The figure shows three views and two pictorial views of one solid part (mm, origin at its lowest corner). Answer the questions. Coordinates: 2 decimals unless noted, no trailing zeros. Write each loop counter-clockwise with the first axis right and the second up, starting at its lowest first coordinate (ties: lowest second). Pieces come first, ordered by that corner, then holes. Notation, with made-up numbers: M 70.5,85.5 L 99.5,85.5 A14 ccw 99.5,108.5 Z; hole C 81.5,-36 d10. An arc over 180 degrees is marked long. Write item = value, one per line.
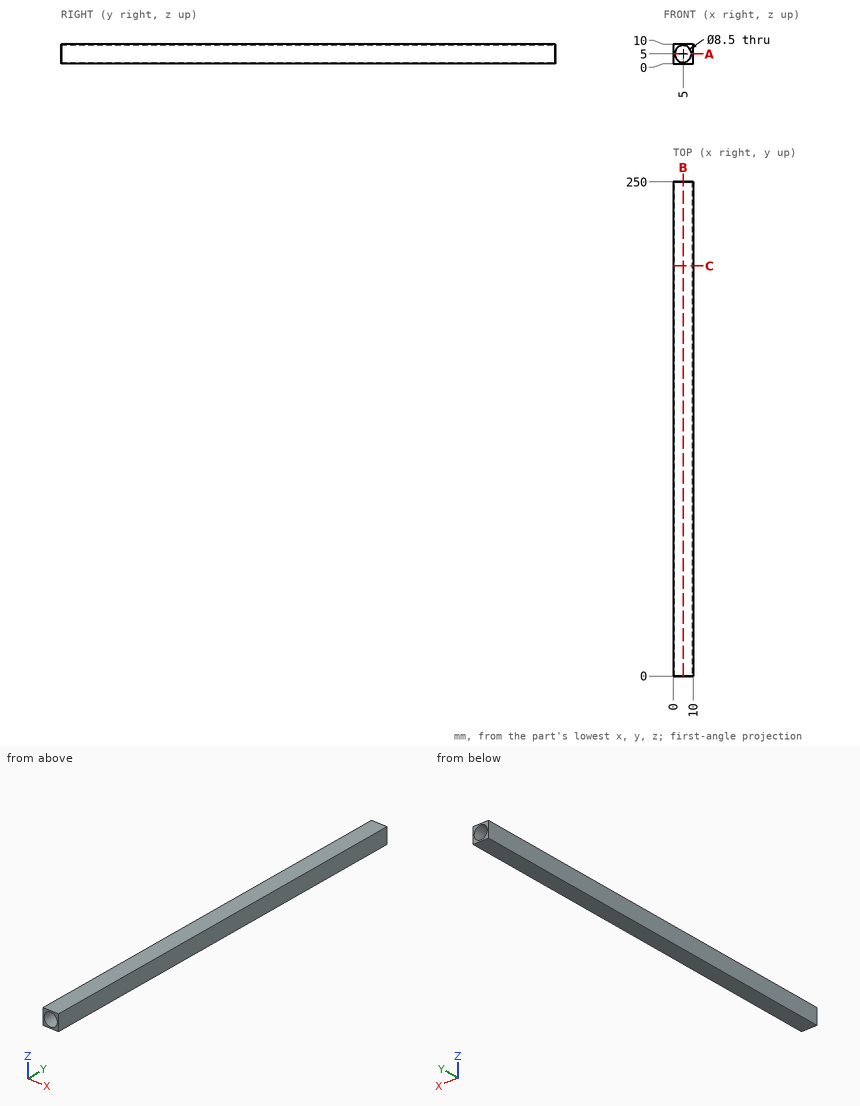
Item 1: Consider line 1 along Z through (x, y) = (5.5, 35); line 2 along X through (y, z) = (232, 8.5); line 3 along Z through (x, y) = (3.75, 213). Determine where each line is inside the solid, lowest interval first. Write a range as from..to.
Worked answers:
line_1 = 0..0.78, 9.22..10
line_2 = 0..2.59, 7.41..10
line_3 = 0..0.94, 9.06..10
Item 2: Find section B-B (x = 5). Determine the outline of the cut face in (y, z), and give its area (3 significant figures).
Worked answers:
outline = M 0,0 L 250,0 L 250,0.75 L 0,0.75 Z; M 0,9.25 L 250,9.25 L 250,10 L 0,10 Z
area = 375 mm²
Item 3: Find section C-C (y = 207.5). Determine the outline of the cut face in (x, z).
Worked answers:
outline = M 0,0 L 10,0 L 10,10 L 0,10 Z; hole C 5,5 d8.5
Item 4: Find section A-A (z = 5). Determine the outline of the cut face in (x, y), and give its area (3 significant figures).
Worked answers:
outline = M 0,0 L 0.75,0 L 0.75,250 L 0,250 Z; M 9.25,0 L 10,0 L 10,250 L 9.25,250 Z
area = 375 mm²
